Geometry: final body of the model. Coordinates: model frame, mm. A direction names the side the tool comes from. Give positions to 0.01 mm unless a question says otherwise; leave off trailing zeros. Write each loop counter-clockwise with the first axis right and the second up, starting at its lowest first coordinate (ties: lowest second). Pieces come first, ordered by that corner, then holes. Notation, with made-up numbers: (58.5, 4) - (105.5, 4) arc R18 cw to (105.5, 29) - close; hole circle Ø10 at (19.5, 21). An arc over 180 degrees is marked (long way). One line per question, with ' | ' between items. Start each with the question number.
```python
from build123d import *

# Parameters (mm, degrees)
SKETCH_1_W          = 88
SKETCH_1_H          = 68
EXTRUDE_1_DEPTH     = 37
SKETCH_2_W          = 52
SKETCH_2_H          = 113
EXTRUDE_2_DEPTH     = 60
SKETCH_3_R          = 5
CUT_EXTRUDE_1_DEPTH = 60
CUT_EXTRUDE_2_DEPTH = 23
SKETCH_5_OUTSIDE_W  = 121.056
SKETCH_5_OUTSIDE_H  = 146.056
CUT_EXTRUDE_3_DEPTH = 38
SKETCH_7_W          = 52
SKETCH_7_H          = 34
SKETCH_7_H_2        = 11
EXTRUDE_3_DEPTH     = 30
FILLET_1_R          = 8
SKETCH_8_W          = 32
SKETCH_8_H          = 30
EXTRUDE_4_DEPTH     = 5
SKETCH_9_R          = 14
EXTRUDE_5_DEPTH     = 10
EXTRUDE_6_DEPTH     = 8
FILLET_2_R          = 5
EXTRUDE_7_DEPTH     = 8
SKETCH_12_R         = 6
EXTRUDE_8_DEPTH     = 8


with BuildPart() as part:
    # 草图1 → 凸台-拉伸1 (new body)
    with BuildSketch(Plane.XY):
        Rectangle(SKETCH_1_W, SKETCH_1_H)
    extrude(amount=EXTRUDE_1_DEPTH)

    # 草图2 → 凸台-拉伸2 (add)
    with BuildSketch(Plane.XY.offset(37)):
        with Locations((0, 11.5)):
            Rectangle(SKETCH_2_W, SKETCH_2_H)
    extrude(amount=-EXTRUDE_2_DEPTH)

    # 草图3 → 切除-拉伸1 (cut)
    with BuildSketch(Plane(origin=(0, 0, -23), x_dir=(-1, 0, 0), z_dir=(0, 0, -1))):
        with Locations((-33.35, 21.45)):
            Circle(SKETCH_3_R)
        with Locations((33.35, 21.45)):
            Circle(SKETCH_3_R)
        with Locations((33.35, -21.45)):
            Circle(SKETCH_3_R)
        with Locations((-33.35, -21.45)):
            Circle(SKETCH_3_R)
    extrude(amount=-CUT_EXTRUDE_1_DEPTH, mode=Mode.SUBTRACT)

    # 草图4 → 切除-拉伸2 (cut)
    with BuildSketch(Plane(origin=(0, 0, -23), x_dir=(-1, 0, 0), z_dir=(0, 0, -1))):
        with BuildLine():
            Line((-26, 29.63397825), (-26, 13.26602175))
            ThreePointArc((-26, 13.26602175), (-22.35, 21.45), (-26, 29.63397825))
        make_face()
        with BuildLine():
            Line((26, 29.63397825), (26, 13.26602175))
            ThreePointArc((26, 13.26602175), (22.35, 21.45), (26, 29.63397825))
        make_face()
        with BuildLine():
            Line((26, -13.26602175), (26, -29.63397825))
            ThreePointArc((26, -29.63397825), (22.35, -21.45), (26, -13.26602175))
        make_face()
        with BuildLine():
            Line((-26, -13.26602175), (-26, -29.63397825))
            ThreePointArc((-26, -29.63397825), (-22.35, -21.45), (-26, -13.26602175))
        make_face()
    extrude(amount=-CUT_EXTRUDE_2_DEPTH, mode=Mode.SUBTRACT)

    # 草图5 outside → 切除-拉伸3 (cut, through all)
    with BuildSketch(Plane(origin=(0, 0, 0), x_dir=(-1, 0, 0), z_dir=(0, 0, -1))):
        with Locations((0, 11.5)):
            Rectangle(SKETCH_5_OUTSIDE_W, SKETCH_5_OUTSIDE_H)
        with BuildLine():
            Line((-34, 34), (34, 34))
            ThreePointArc((34, 34), (41.071067812, 31.071067812), (44, 24))
            Line((44, 24), (44, -24))
            ThreePointArc((44, -24), (41.071067812, -31.071067812), (34, -34))
            Line((34, -34), (-34, -34))
            ThreePointArc((-34, -34), (-41.071067812, -31.071067812), (-44, -24))
            Line((-44, -24), (-44, 24))
            ThreePointArc((-44, 24), (-41.071067812, 31.071067812), (-34, 34))
        make_face(mode=Mode.SUBTRACT)
    extrude(amount=-CUT_EXTRUDE_3_DEPTH, mode=Mode.SUBTRACT)

    # 草图7 → 凸台-拉伸3 (add)
    with BuildSketch(Plane.XY):
        with Locations((0, 51)):
            Rectangle(SKETCH_7_W, SKETCH_7_H)
        with Locations((0, -39.5)):
            Rectangle(SKETCH_7_W, SKETCH_7_H_2)
    extrude(amount=EXTRUDE_3_DEPTH)

    # 圆角1
    fillet_1_edges = [part.edges().sort_by_distance(p)[0] for p in [
        (-26, -45, 3.5),
        (26, 68, 3.5),
        (-26, 68, 3.5),
        (26, -45, 3.5),
    ]]
    fillet(fillet_1_edges, radius=FILLET_1_R)

    # 草图8 → 凸台-拉伸4 (add)
    with BuildSketch(Plane(origin=(0, 0, -23), x_dir=(-1, 0, 0), z_dir=(0, 0, -1))):
        with Locations((0, 51)):
            Rectangle(SKETCH_8_W, SKETCH_8_H)
    extrude(amount=EXTRUDE_4_DEPTH)

    # 草图9 → 凸台-拉伸5 (add)
    with BuildSketch(Plane(origin=(0, 0, -28), x_dir=(-1, 0, 0), z_dir=(0, 0, -1))):
        with Locations((0, 51)):
            Circle(SKETCH_9_R)
    extrude(amount=EXTRUDE_5_DEPTH)

    # 草图10 → 凸台-拉伸6 (add)
    with BuildSketch(Plane(origin=(0, 0, -38), x_dir=(-1, 0, 0), z_dir=(0, 0, -1))):
        Polygon((-6.149615956, 61.651447283), (-12.299231913, 51), (-6.149615956, 40.348552717), (6.149615956, 40.348552717), (12.299231913, 51), (6.149615956, 61.651447283), align=None)
    extrude(amount=EXTRUDE_6_DEPTH)

    # 圆角2
    fillet_2_edges = [part.edges().sort_by_distance(p)[0] for p in [
        (16, 66, -25.5),
        (16, 36, -25.5),
        (-16, 36, -25.5),
        (-16, 66, -25.5),
    ]]
    fillet(fillet_2_edges, radius=FILLET_2_R)

    # 草图11 → 凸台-拉伸7 (add)
    with BuildSketch(Plane(origin=(0, 0, -46), x_dir=(-1, 0, 0), z_dir=(0, 0, -1))):
        Polygon((0, 42.898459123), (7.016140209, 46.949229562), (7.016140209, 55.050770438), (0, 59.101540877), (-7.016140209, 55.050770438), (-7.016140209, 46.949229562), align=None)
    extrude(amount=EXTRUDE_7_DEPTH)

    # 草图12 → 凸台-拉伸8 (add)
    with BuildSketch(Plane(origin=(0, 0, -54), x_dir=(-1, 0, 0), z_dir=(0, 0, -1))):
        with Locations((0, 51)):
            Circle(SKETCH_12_R)
    extrude(amount=EXTRUDE_8_DEPTH)


solid = part.part
```
1) First-contact query: pin 1 Ø3 at (x, y) = (16.5, 55) entering from +Z; pin 2 Ø6 at (x, y) = (33.5, -29.5) entering from -Z; pin 3 Ø2.5 at (y, z) = (52.5, -50.5) entering from -X. Flat tips, straight axial feed; report the tip coordinate or a pass-through.
2) Pull-direction query (Y, two-part tool) for faces 6 (the cylindrical face through (23.719, -42.594, 3.129)), 7 (the cylindrical face through (-22.35, 21.32, -11.66)), 8 (the cylindrical face through (-23.719, 65.594, 3.129)); classes: +Y half, -Y half, draft (parallel to the pull), parting line (faces both ways), or undercut.
3) Section D-D, the plane x = -3.5. Output: boundary loops of the cut face in (y, z).
4) Line query: L1, parallel to Y at x = 33, z = 18; L2, parallel to Z at x = 15.5, y = 14.5; L3, parallel to X at y = 46.5, z = -33.5. Output: solid intervals per line, ascending.
5) Section B-B, the plane z = 7. Output: boundary loops of the cut face in (x, y).
6) Reachability of faces 1 (the flat face through (3.459, 57.105, -49.944)), 2 (the flat face through (0, 61.651, -42)), 3 (the cylindrical face through (-15, 38, -26)), 4 (the flat face through (4, 46, -54)), 5 (the flat face through (7.016, 51, -50)) from +Z, -Z, +X, -X, +Y, -Y: full face, straight path, thin tool, end or side. Return the list, or none.
7) Section C-C, the plane y = 6. Output: boundary loops of the cut face in (x, z), plus the area to 3 significant figures.
8) Section A-A, the plane y = -21.45. Output: boundary loops of the cut face in (x, z).
Answer key:
1) pin 1: z = 30 | pin 2: z = 0 | pin 3: x = -7.02
2) face 6: -Y half | face 7: undercut | face 8: +Y half
3) outline: (-45, -23) - (36, -23) - (36, -28) - (37.44, -28) - (37.44, -38) - (40.35, -38) - (40.35, -46) - (44.92, -46) - (44.92, -54) - (46.13, -54) - (46.13, -62) - (55.87, -62) - (55.87, -54) - (57.08, -54) - (57.08, -46) - (61.65, -46) - (61.65, -38) - (64.56, -38) - (64.56, -28) - (66, -28) - (66, -23) - (68, -23) - (68, 30) - (34, 30) - (34, 37) - (-34, 37) - (-34, 30) - (-45, 30) - close
4) L1: -34 to -26.44, -16.46 to 16.46, 26.44 to 34 | L2: -23 to 37 | L3: -13.26 to 13.26
5) outline: (-44, -24) arc R10 ccw to (-34, -34) - (-26, -34) - (-26, -37) arc R8 ccw to (-18, -45) - (18, -45) arc R8 ccw to (26, -37) - (26, -34) - (34, -34) arc R10 ccw to (44, -24) - (44, 24) arc R10 ccw to (34, 34) - (26, 34) - (26, 60) arc R8 ccw to (18, 68) - (-18, 68) arc R8 ccw to (-26, 60) - (-26, 34) - (-34, 34) arc R10 ccw to (-44, 24) - close; hole circle Ø10 at (-33.35, -21.45); hole circle Ø10 at (-33.35, 21.45); hole circle Ø10 at (33.35, -21.45); hole circle Ø10 at (33.35, 21.45)
6) face 1: -Z, +X, +Y | face 2: -Z, +X, -X, +Y | face 3: -Z, -X, -Y | face 4: -Z | face 5: -Z, +X, +Y, -Y
7) outline: (-44, 0) - (-26, 0) - (-26, -23) - (26, -23) - (26, 0) - (44, 0) - (44, 37) - (-44, 37) - close | area: 4,450 mm^2
8) outline: (-44, 0) - (-38.35, 0) - (-38.35, 37) - (-44, 37) - close; (-28.35, 0) - (-22.35, 0) - (-22.35, -23) - (22.35, -23) - (22.35, 0) - (28.35, 0) - (28.35, 37) - (-28.35, 37) - close; (38.35, 0) - (44, 0) - (44, 37) - (38.35, 37) - close
